Design review of the part built by this model. Coordinates are the model's own, in mm. Face numbers are marked on the shaded views. A direction names the side the tool comes from. Round coordinates to 2 decimals unless told otherwise and drop trailing zeros. Order: outer loops, then holes, each group sorted by start corner. A loop starts at its lowest first (then second) coordinate and runs counter-clockwise, first axis right, second up. Notation, with made-up numbers: M 69.5,44.5 L 87.5,44.5 A24 cw 87.5,66.5 Z; hole C -9.5,24.25 d8. An arc over 180 degrees is marked long. Use a Markdown table: item, result. Add a question column.
(1) Take a section at B-B (z = -35). Write out the cut boundary in (x, y), then the cut area to 3 significant figures.
(2) Take a section at D-D (y = -10). Write out the cut boundary in (x, z) (3 decimals), then the cut area to 3 significant figures.
(3) Take a section at A-A (x = 35). Write out the cut boundary in (y, z) (3 decimals), then the cut area to 3 significant figures.
(4) Take a section at C-C (z = 6). Write out the cut boundary in (x, y).
(5) For pin 1 (6 mm diameter, centred on y = -11.5, z = -17.5, fed in from -X); pin 2 (7.5 mm diameter, centred on x = -20, y = -16, fed in from +Z), all flat-tipped, find the tip position at first contact; note any pin that passes through.
(6) Machinability: for the marked faces 1 and 2, which of the approach directions +Z, -Z, +X, -X, +Y, -Y give a long, thin tool a straight path to every point of the face, cutting with its end or side? Answer none if there is none.
(7) To check wall thickness, follow probe 1 along Y at (x, z) = (34.5, 39); probe 2 along Z at (x, y) = (7.5, -15) (3 decimals); probe 3 along X at (y, z) = (-2, 2.5). State the ranges of each line that lie inside material, in increasing order. Write a range as from..to.
```python
from build123d import *

# Parameters (mm, degrees)
F1_DEPTH = 6.35
F2_R     = 50.8
F3_W     = 118.5620874166
F3_H     = 5.6165596008
F4_DEPTH = 25.4


with BuildPart() as f1:
    # F0 (on Front) → F1 (new body)
    with BuildSketch(Plane.XZ):
        Polygon((-59.2810437083, -53.975), (0, -53.975), (59.2810437083, -53.975), (59.2810437083, 53.975), (-59.2810437083, 53.975), align=None)
        with BuildLine():
            ThreePointArc((-50.9875, 3.0062948354), (-51.3975505063, 2.0163453417), (-52.3875, 1.6062948354))
            ThreePointArc((-52.3875, 1.6062948354), (-53.3774494937, 3.996244329), (-50.9875, 3.0062948354))
        make_face(mode=Mode.SUBTRACT)
        with BuildLine():
            ThreePointArc((-42.545, 0), (0, 42.545), (42.545, 0))
            ThreePointArc((42.545, 0), (30.0838580056, -30.0838580056), (0, -42.545))
            ThreePointArc((0, -42.545), (-30.0838580056, -30.0838580056), (-42.545, 0))
        make_face(mode=Mode.SUBTRACT)
        with BuildLine():
            ThreePointArc((53.7845, 3.1811562367), (53.3753281733, 2.1933280634), (52.3875, 1.7841562367))
            ThreePointArc((52.3875, 1.7841562367), (51.3996718267, 4.16898441), (53.7845, 3.1811562367))
        make_face(mode=Mode.SUBTRACT)
    extrude(amount=F1_DEPTH)

    # F2
    f2_edges = [f1.edges().sort_by_distance(p)[0] for p in [
        (59.281044, -3.175, 53.975),
        (-59.281044, -3.175, 53.975),
    ]]
    fillet(f2_edges, radius=F2_R)

    # F3 (on face) → F4 (join)
    with BuildSketch(Plane.XZ.offset(6.35)):
        with Locations((0, -51.1667201996)):
            Rectangle(F3_W, F3_H)
    extrude(amount=F4_DEPTH)


solid = f1.part
```
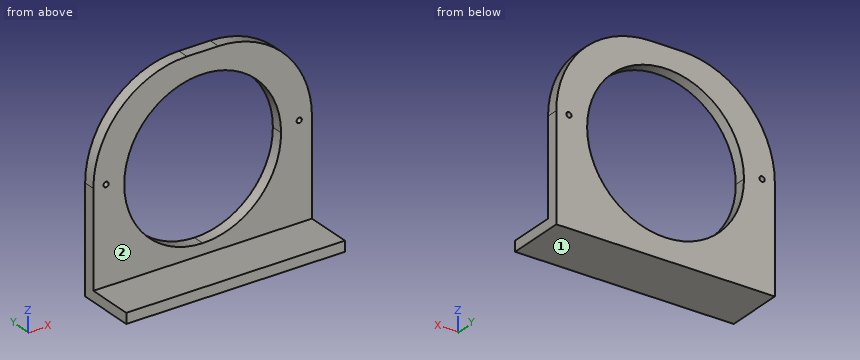
Verdict:
| question | item | result |
|---|---|---|
| 1 | outline | M -59.28,-6.35 L -24.19,-6.35 L -24.19,0 L -59.28,0 Z; M 24.19,-6.35 L 59.28,-6.35 L 59.28,0 L 24.19,0 Z |
| 1 | area | 446 mm^2 |
| 2 | outline | M -59.281,-53.975 L 59.281,-53.975 L 59.281,-48.358 L -59.281,-48.358 Z |
| 2 | area | 666 mm^2 |
| 3 | outline | M -31.75,-53.975 L 0,-53.975 L 0,-24.188 L -6.35,-24.188 L -6.35,-48.358 L -31.75,-48.358 Z; M -6.35,24.188 L 0,24.188 L 0,46.504 L -6.35,46.504 Z |
| 3 | area | 474 mm^2 |
| 4 | outline | M -59.2,-6.35 L -42.12,-6.35 L -42.12,0 L -59.2,0 Z; M 42.12,-6.35 L 59.2,-6.35 L 59.2,0 L 42.12,0 Z |
| 5 | pin 1 | passes through |
| 5 | pin 2 | stops at z = -48.36 |
| 6 | face 1 | -Z, +X, -X, +Y, -Y |
| 6 | face 2 | +Z, +X, -X, -Y |
| 7 | probe 1 | y = -6.35..0 |
| 7 | probe 2 | z = -53.975..-48.358 |
| 7 | probe 3 | x = -59.28..-53.69, -51.08..-42.47, 42.47..51.17, 53.61..59.28 |
